Geometry check sheet. Reference: drawing and pictorial views, mm from the part's lowest x, y, z. A direction names the side the tool comes from. Round coordinates to 2 decimals unless told otherwise and drop trailing zeros. Loops run counter-clockwise (first coordinate to the right, second up) from the corner with the lowest first, then second, coordinate; pieces in that order, holes last. Notation, with made-up numbers: (72, -24) -> (131, -24) arc R14 cw to (131, -3) -> close; hole circle Ø6 at (18, -30.5). An arc over 180 degrees is marked (long way). Write item = value, one per line.
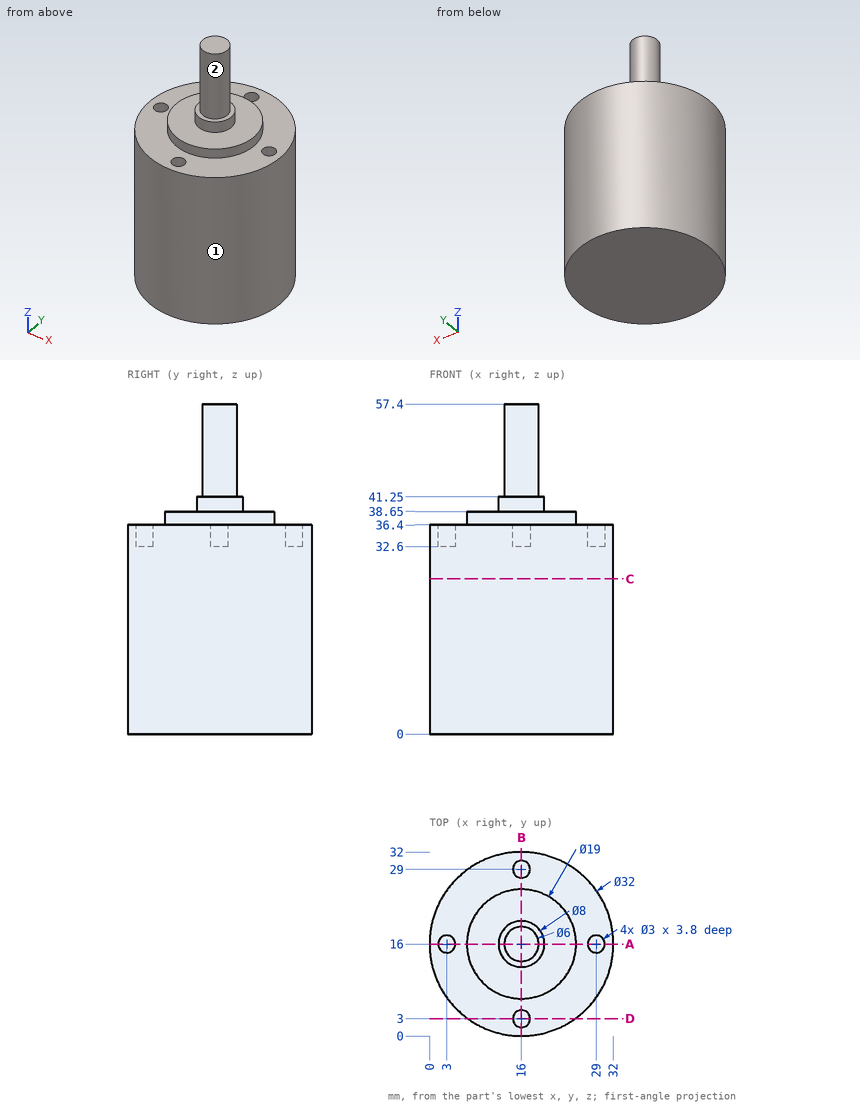
(1) Sectioned sample at C-C, the plane z = 27. Record the cut outline in (x, y), and give its area (3 significant figures).
Filled sheet:
outline = circle Ø32 at (16, 16)
area = 804 mm2
(2) Sectioned sample at D-D, the plane y = 3. Record the cut outline in (x, z).
Filled sheet:
outline = (6.67, 0) -> (25.33, 0) -> (25.33, 36.4) -> (17.5, 36.4) -> (17.5, 32.6) -> (14.5, 32.6) -> (14.5, 36.4) -> (6.67, 36.4) -> close
(3) Material ranges on probe 1 along Y at (x, z) = (16, 34.5); probe 2 along Y at (x, z) = (3, 34.35); probe 3 along Z at (x, y) = (20, 24.5), recorded low to high. Write a range as from..to.
Filled sheet:
probe_1 = 0..1.5, 4.5..27.5, 30.5..32
probe_2 = 6.67..14.5, 17.5..25.33
probe_3 = 0..38.65
(4) Sectioned sample at A-A, the plane y = 16. Record the cut outline in (x, z), and give its area (3 significant figures).
Filled sheet:
outline = (0, 0) -> (32, 0) -> (32, 36.4) -> (30.5, 36.4) -> (30.5, 32.6) -> (27.5, 32.6) -> (27.5, 36.4) -> (25.5, 36.4) -> (25.5, 38.65) -> (20, 38.65) -> (20, 41.25) -> (19, 41.25) -> (19, 57.4) -> (13, 57.4) -> (13, 41.25) -> (12, 41.25) -> (12, 38.65) -> (6.5, 38.65) -> (6.5, 36.4) -> (4.5, 36.4) -> (4.5, 32.6) -> (1.5, 32.6) -> (1.5, 36.4) -> (0, 36.4) -> close
area = 1,300 mm2
(5) Set-up check for the marked faces 1 and 2: record each of +Z, -Z, +X, -X, +Y, -Y from which the full face is reachable in a straight line by a thin tool's end or side.
Filled sheet:
face_1 = +Z, -Z
face_2 = +Z
(6) Go/stop test with flat-tipped pins: pin 1 Ø1.8 at (x, y) = (29, 16) entering from +Z; pin 2 Ø2.5 at (x, y) = (15.5, 28.5) entering from +Z; pin 3 Ø2 at (y, z) = (5.5, 34) entering from -X. Record where each tip stops, or that it passes through.
Filled sheet:
pin_1 = 32.6
pin_2 = 36.4
pin_3 = 3.13
